The model under review builds one solid part; all positions refer to its coordinate system, in mm. Coordinates: 2 decimals unless noted, no trailing zeros. Order: outer loops, then holes, each group sorted by start corner. A loop starts at its lowest first (then second) coordinate and runs counter-clockwise, first axis right, second up.
Autodesk Inventor part; units mm, degrees
ref_plane "YZ Plane" through (0, 0, 0) normal (1, 0, 0) x (0, 1, 0)
ref_plane "XZ Plane" through (0, 0, 0) normal (0, 1, 0) x (-1, 0, 0)
ref_plane "XY Plane" through (0, 0, 0) normal (0, 0, 1) x (1, 0, 0)
sketch "Эскиз1" plane through (0, 0, 0) normal (0, 0, 1) x (1, 0, 0)
  line L0 (0, 0) -> (-10, 0)
  line L1 (-10, 0) -> (-10, 10)
  line L2 (-10, 10) -> (0, 10)
  line L3 (0, 10) -> (0, 0)
  dimension "d0" = 10
  dimension "d1" = 10
extrude "Выдавливание1" add sketch "Эскиз1" along normal blind 210
sketch "Эскиз2" plane through (0, 0, 210) normal (0, 0, 1) x (1, 0, 0)
  line L0 (-10, 10) -> (-10, 0)
  line L1 (0, 0) -> (0, 10)
  line L2 (-10, 3) -> (0, 3)
  line L3 (0, 3) -> (0, 7)
  line L4 (0, 7) -> (-10, 7)
  line L5 (-10, 7) -> (-10, 3)
  line L6 (-10, 5) -> (0, 5)
  point P0 (0, 3)
  dimension "d4" = 4
extrude "Выдавливание2" add sketch "Эскиз2" along normal blind 4
sketch "Эскиз3" plane through (0, 0, 0) normal (0, 0, -1) x (-1, 0, 0)
  line L0 (10, 7) -> (10, 3)
  line L1 (0, 0) -> (0, 3)
  line L2 (10, 7) -> (0, 7)
  line L3 (0, 7) -> (0, 3)
  line L4 (0, 3) -> (10, 3)
  line L5 (10, 3) -> (10, 7)
extrude "Выдавливание3" add sketch "Эскиз3" along normal blind 4
sketch "Эскиз4" plane through (-10, 0, 0) normal (0, -1, 0) x (1, 0, 0)
  line L0 (10, 0) -> (10, 210)
  line L1 (10, 105) -> (0, 105)
  line L2 (0, 0) -> (0, 210)
  line L3 (5, 105) -> (5, 0)
  line L4 (0, 0) -> (10, 0)
  line L5 (6.7537, 95) -> (3.2463, 95)
  line L6 (3.2463, 95) -> (3.2463, 85)
  line L7 (3.2463, 85) -> (6.7537, 85)
  line L8 (6.7537, 85) -> (6.7537, 95)
  line L9 (7.0866, 70) -> (2.9134, 70)
  line L10 (2.9134, 70) -> (2.9134, 60)
  line L11 (2.9134, 60) -> (7.0866, 60)
  line L12 (7.0866, 60) -> (7.0866, 70)
  line L13 (7.0866, 45) -> (2.9134, 45)
  line L14 (2.9134, 45) -> (2.9134, 35)
  line L15 (2.9134, 35) -> (7.0866, 35)
  line L16 (7.0866, 35) -> (7.0866, 45)
  line L17 (6.7537, 20) -> (3.2463, 20)
  line L18 (3.2463, 20) -> (3.2463, 10)
  line L19 (3.2463, 10) -> (6.7537, 10)
  line L20 (6.7537, 10) -> (6.7537, 20)
  dimension "d9" = 10
  dimension "d10" = 10
  dimension "d11" = 10
  dimension "d12" = 10
  dimension "d13" = 10
  dimension "d14" = 15
  dimension "d15" = 15
  dimension "d16" = 15
extrude "Выдавливание4" add sketch "Эскиз4" along normal blind 4 contours L19 L18 L17 L3 | L3 L17 L20 L19 | L5 L8 L7 L3 | L3 L7 L6 L5 | L15 L14 L13 L3 | L3 L13 L16 L15 | L9 L12 L11 L3 | L3 L11 L10 L9
sketch "Эскиз5" plane through (-10, 10, 0) normal (0, 1, 0) x (1, 0, 0)
  line L0 (9, -52.1164) -> (1, -52.1164)
  line L1 (1, -52.1164) -> (1, -72.1164)
  line L2 (1, -72.1164) -> (9, -72.1164)
  line L3 (9, -72.1164) -> (9, -52.1164)
  point P0 (10, 0)
  point P1 (10, -52.1164)
  dimension "d19" = 8
  dimension "d20" = 20
  dimension "d21" = 1
extrude "Выдавливание5" add sketch "Эскиз5" along normal blind 8
fillet "Сопряжение1" radius 2 2 edges at (-1, 18, 62.1164) (-9, 18, 62.1164)
sketch "Эскиз6" plane through (-1, 10, 52.1164) normal (0, 0, -1) x (-1, 0, 0)
  line L0 (2, 8) -> (6, 8)
  line L1 (8, 0) -> (8, 6)
  circle A0 centre (4, 3) radius 1.5
  point P0 (-1, -10)
  point P1 (4, 8)
  point P2 (8, 3)
  dimension "d25" = 3
extrude "Выдавливание6" add sketch "Эскиз6" along normal blind 50
properties part number "центр пушки"
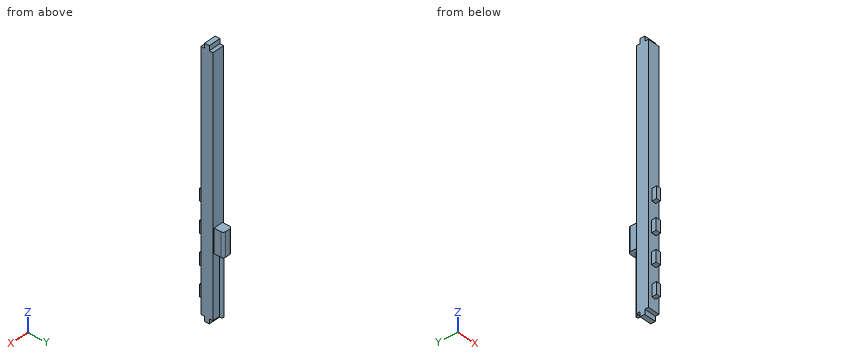
(1) For pin 1 Ø1.5 at (y, z) = (13.5, 26) entering from -X; pin 2 Ø1.2 at (x, z) = (-5, 211.5) entering from +Y; pin 3 Ø2 at (y, z) = (-2.5, 15.5) entering from -X, all flat-tipped, find the tip position at first contact; note any pin that passes through.
A:
pin 1: stops at x = -6.5
pin 2: stops at y = 7
pin 3: stops at x = -6.75
(2) Wall thickness on probe 1 along Y at (x, z) = (-3.25, 79.5); probe 2 along Z at (x, y) = (-4.5, 1); probe 3 along Z at (x, y) = (-2.75, 15.5): over which ranges is each line inside the solid? List them lowest first.
A:
probe 1: y = 0 to 10
probe 2: z = 0 to 210
probe 3: z = 52.12 to 72.12
(3) We need section A-A, the plane z = 79. Write out the cut boundary in (x, y), and give its area (3 significant figures).
A:
outline: (-10, 0) - (0, 0) - (0, 10) - (-10, 10) - close
area: 100 mm2
